Work out the finished part from the listing and answer in its coordinate system (mm). A direction names the side the tool comes from. Coordinates: 2 decimals unless noted, no trailing zeros. Loops run counter-clockwise (first coordinate to the right, second up) from the corner with the lowest first, then second, coordinate; pieces in that order, holes last.
```python
from build123d import *

# Parameters (mm, degrees)
SKETCH1_R           = 12.5
BOSS_EXTRUDE1_DEPTH = 5
SKETCH2_R           = 2.5
BOSS_EXTRUDE2_DEPTH = 60
BOSS_EXTRUDE3_DEPTH = 5
REVOLVE1_ANGLE      = 15
SKETCH7_R           = 7.5
BOSS_EXTRUDE4_DEPTH = 5
CIRPATTERN1_COUNT   = 6
FILLET1_R           = 3
SKETCH8_R           = 7.5
BOSS_EXTRUDE5_DEPTH = 10
BOSS_EXTRUDE5_TAPER = 30


with BuildPart() as part:
    # Sketch1 → Boss-Extrude1 (new body)
    with BuildSketch(Plane(origin=(0, 0, 0), x_dir=(1, 0, 0), z_dir=(0, 1, 0))):
        Circle(SKETCH1_R)
    extrude(amount=BOSS_EXTRUDE1_DEPTH)

    # Sketch2 → Boss-Extrude2 (add)
    with BuildSketch(Plane(origin=(0, 5, 0), x_dir=(1, 0, 0), z_dir=(0, 1, 0))):
        Circle(SKETCH2_R)
    extrude(amount=BOSS_EXTRUDE2_DEPTH)

    # Sketch3 → Boss-Extrude3 (add)
    with BuildSketch(Plane(origin=(0, 65, 0), x_dir=(1, 0, 0), z_dir=(0, 1, 0))):
        with BuildLine():
            Line((2.5, 0), (12.5, 0))
            ThreePointArc((12.5, 0), (12.074072829, -3.235238064), (10.825317547, -6.25))
            Line((10.825317547, -6.25), (2.165063509, -1.25))
            ThreePointArc((2.165063509, -1.25), (-0.647047613, -2.414814566), (-2.5, 0))
            Line((-2.5, 0), (-12.5, 0))
            ThreePointArc((-12.5, 0), (-12.074072829, 3.235238064), (-10.825317547, 6.25))
            Line((-10.825317547, 6.25), (-2.165063509, 1.25))
            ThreePointArc((-2.165063509, 1.25), (0.647047613, 2.414814566), (2.5, 0))
        make_face()
    extrude(amount=-BOSS_EXTRUDE3_DEPTH)

    # Sketch6 → Revolve1 (revolve)
    with BuildSketch(Plane.XY):
        Polygon((8, 5), (3.5, 32.491106736), (7.5, 59.982213472), (0, 59.982213472), (0, 5), align=None)
    revolve1 = revolve(axis=Axis((0, 5, 0), (0, 1, 0)), revolution_arc=REVOLVE1_ANGLE)

    # Sketch7 → Boss-Extrude4 (add)
    with BuildSketch(Plane(origin=(0, 65, 0), x_dir=(1, 0, 0), z_dir=(0, 1, 0))):
        Circle(SKETCH7_R)
    extrude(amount=-BOSS_EXTRUDE4_DEPTH)

    # CirPattern1: Revolve1 ×6 about axis
    cirpattern1_axis = Axis((0, 0, 0), (0, 1, 0))
    for i in range(1, CIRPATTERN1_COUNT):
        add(revolve1.rotate(cirpattern1_axis, i * 360 / CIRPATTERN1_COUNT))

    # Fillet1
    fillet1_edges = [part.edges().sort_by_distance(p)[0] for p in [
        (-12.5, 5, 0),
    ]]
    fillet(fillet1_edges, radius=FILLET1_R)

    # Sketch8 → Boss-Extrude5 (add)
    with BuildSketch(Plane(origin=(0, 60, 0), x_dir=(-1, 0, 0), z_dir=(0, -1, 0))):
        Circle(SKETCH8_R)
    extrude(amount=BOSS_EXTRUDE5_DEPTH, taper=BOSS_EXTRUDE5_TAPER)


solid = part.part
```
1. A cutting plane is placed at A-A, the plane x = 0. Give the vertices of the cut face in (y, z).
2. A cutting plane is placed at C-C, the plane y = 48. Give the vertices of the cut face in (x, z).
3. Straight lines are drawn through the part: probe 1 along X at (y, z) = (13, -4.75); probe 2 along Y at (x, z) = (5.5, 7); probe 3 along X at (y, z) = (10, 4.5). For each, find the intervals that lie inside material, in ascending order.
4. A cutting plane is placed at B-B, the plane y = 37.5. Give the vertices of the cut face in (x, z).
5. For faces 1 (the flat face through (1.99, 26.77, -3.45)), 2 (the flat face through (1.99, 26.77, 3.45)), 3 (the flat face through (-1.99, 26.77, -3.45)), 4 (the conical face through (-5.482, 46.429, 0.712)), determine the directions among +Z, -Z, +X, -X, +Y, -Y from which every point of the face is accessible in a straight line to the end or side of a thin tool.
6. Determine the mould class of faces 5 (the cylindrical face through (2.304, 27.845, 0.969)), 6 (the conical face through (2.125, 46.429, -5.103)), 7 (the conical face through (-5.67, 18.94, 0.74)) for opening direction Z: released by +Z, released by -Z, zero draft, split by the parting line, or undercut.
7. Each of these flat-tipped pins is pushed along its axis until it touches: P1, Ø1.5, axis at x = -10.5, y = 63, coming from the +Z side; P2, Ø10, axis at y = 25.5, z = -6, coming from the +X side; P3, Ø6, axis at x = -4.5, y = 36, coming from the -Z side. Where does it stop, or does it pass through?
Answers below:
1. outline: (0, -12.5) - (2, -12.5) arc R3 ccw to (5, -9.5) - (5, -2.5) - (51.34, -2.5) - (60, -7.5) - (65, -7.5) - (65, 7.5) - (60, 7.5) - (51.34, 2.5) - (5, 2.5) - (5, 9.5) arc R3 ccw to (2, 12.5) - (0, 12.5) - close
2. outline: (-5.76, 0) - (-2.5, 0) arc R2.5 ccw to (-1.77, -1.77) - (-4.07, -4.07) arc R5.76 ccw to (-2.88, -4.99) - (-1.25, -2.17) arc R2.5 ccw to (0.65, -2.41) - (1.49, -5.56) arc R5.76 ccw to (2.88, -4.99) - (1.25, -2.17) arc R2.5 ccw to (2.41, -0.65) - (5.56, -1.49) arc R5.76 ccw to (5.76, 0) - (2.5, 0) arc R2.5 ccw to (1.77, 1.77) - (4.07, 4.07) arc R5.76 ccw to (2.88, 4.99) - (1.25, 2.17) arc R2.5 ccw to (-0.65, 2.41) - (-1.49, 5.56) arc R5.76 ccw to (-2.88, 4.99) - (-1.25, 2.17) arc R2.5 ccw to (-2.41, 0.65) - (-5.56, 1.49) arc R5.76 ccw to start
3. probe 1: x = -4.71 to -2.74, 1.27 to 2.74
3. probe 2: y = 0 to 5
3. probe 3: x = -2.6 to -1.21, 2.6 to 4.5
4. outline: (-4.23, 0) - (-2.5, 0) arc R2.5 ccw to (-1.77, -1.77) - (-2.99, -2.99) arc R4.23 ccw to (-2.11, -3.66) - (-1.25, -2.17) arc R2.5 ccw to (0.65, -2.41) - (1.09, -4.08) arc R4.23 ccw to (2.11, -3.66) - (1.25, -2.17) arc R2.5 ccw to (2.41, -0.65) - (4.08, -1.09) arc R4.23 ccw to (4.23, 0) - (2.5, 0) arc R2.5 ccw to (1.77, 1.77) - (2.99, 2.99) arc R4.23 ccw to (2.11, 3.66) - (1.25, 2.17) arc R2.5 ccw to (-0.65, 2.41) - (-1.09, 4.08) arc R4.23 ccw to (-2.11, 3.66) - (-1.25, 2.17) arc R2.5 ccw to (-2.41, 0.65) - (-4.08, 1.09) arc R4.23 ccw to start
5. face 1: +X
5. face 2: +Z
5. face 3: -Z
5. face 4: +Z, -X
6. face 5: undercut
6. face 6: released by -Z
6. face 7: released by +Z
7. P1: stops at z = 0
7. P2: stops at x = 4.74
7. P3: stops at z = -3.71
